Geometry check sheet. Reference: the model listing, model coordinates, mm. Face numbers are marked on the shaded views. A direction names the side the tool comes from. Give positions to 0.01 mm unless a question says otherwise; leave off trailing zeros. Order: outer loops, then holes, each group sorted by start corner. A loop starts at its lowest first (then second) coordinate and runs counter-clockwise, first axis right, second up. Notation, with made-up numbers: M 14.5,35.5 L 57.5,35.5 A32 cw 57.5,70.5 Z; hole C -15.75,30 d4. An arc over 180 degrees is marked long. Put each result on its own line as item: value. Start each with the question number.
Q1. Go/stop test with a flat-tipped pin: pin 1 (0.6 mm diameter, centred on x = 6.5, z = 1, fed in from -Y). Record where the tip stops, or that it passes through.
Q2. Section check B-B on z = 0.6. Record the cut outline in (x, y), then the cut area to 3 significant figures.
Q3. Material ranges on L1, parallel to Y at x = 3, z = 1.2; L2, parallel to X at y = 1.9, z = 0.2; L3, parallel to Z at x = 3.75, y = -0.4, recorded low to high.
Q4. Access from +Z, -Z, +X, -X, +Y, -Y to the whole of each face (thin tool, end or side, straight path). Record for the marked faces 1, 2, 3, 4 and 5.
Q5. Section check D-D on y = 2.45. Record the cut outline in (x, z), then the cut area to 3 significant figures.
Q6. Section check C-C on x = 4. Record the cut outline in (y, z).
Q7. Section check A-A on y = 3.1. Record the cut outline in (x, z).
```python
from build123d import *

# Parameters (mm, degrees)
SKETCH2_W            = 6.3
SKETCH2_H            = 2.6
BOSS_EXTRUDE1_DEPTH  = 1.4
EXTRUDE_THIN2_DEPTH  = 0.4
FILLET1_R            = 0.1
FILLET1_OF_MIRROR3_R = 0.1
MIRROR4_DEPTH        = 0.4
MIRROR4_START        = 2.2
MIRROR4_2_DEPTH      = 0.4
SKETCH4_W            = 0.2
SKETCH4_H            = 0.9
EXTRUDE_THIN3_DEPTH  = 0.2
SKETCH5_W            = 0.2
SKETCH5_H            = 0.9
EXTRUDE_THIN4_DEPTH  = 0.2
SKETCH6_W            = 0.2
SKETCH6_H            = 0.9
EXTRUDE_THIN5_DEPTH  = 0.2
SKETCH8_W            = 1.5
SKETCH8_H            = 1.1
BOSS_EXTRUDE2_DEPTH  = 1.5
FILLET2_R            = 0.2


# Read off the part's stored shape, not the designer's step: Mirror4
with BuildPart() as part:
    # Sketch2 → Boss-Extrude1 (new body)
    with BuildSketch(Plane.XY):
        with Locations((3.15, 1.3)):
            Rectangle(SKETCH2_W, SKETCH2_H)
    extrude(amount=BOSS_EXTRUDE1_DEPTH)

    # Sketch3 → Extrude-Thin2 (add)
    with BuildSketch(Plane.XZ):
        with BuildLine():
            Line((0, 1.4), (0, 0.3))
            ThreePointArc((0, 0.3), (-0.087867966, 0.087867966), (-0.3, 0))
            Line((-0.3, 0), (-0.7, 0))
            Line((-0.7, 0), (-0.7, 0.2))
            Line((-0.7, 0.2), (-0.3, 0.2))
            ThreePointArc((-0.3, 0.2), (-0.229289322, 0.229289322), (-0.2, 0.3))
            Line((-0.2, 0.3), (-0.2, 1.4))
            Line((-0.2, 1.4), (0, 1.4))
        make_face()
    extrude_thin2 = extrude(amount=-EXTRUDE_THIN2_DEPTH)

    # Fillet1
    fillet1_edges = [part.edges().sort_by_distance(p)[0] for p in [
        (-0.2, 0.2, 1.4),
    ]]
    fillet(fillet1_edges, radius=FILLET1_R)

    # Mirror3: Extrude-Thin2 across plane
    add(extrude_thin2.mirror(Plane.ZX.offset(1.3)))

    # Fillet1 of Mirror3
    fillet1_of_mirror3_edges = [part.edges().sort_by_distance(p)[0] for p in [
        (-0.2, 2.4, 1.4),
    ]]
    fillet(fillet1_of_mirror3_edges, radius=FILLET1_OF_MIRROR3_R)

    # Mirror4 outline → Mirror4 (add)
    with BuildSketch(Plane(origin=(0, 0, 0), x_dir=(1, 0, 0), z_dir=(0, 1, 0))):
        with BuildLine():
            Line((7, 0), (6.6, 0))
            ThreePointArc((6.6, 0), (6.387867966, -0.087867966), (6.3, -0.3))
            Line((6.3, -0.3), (6.3, -1.4))
            Line((6.3, -1.4), (6.4, -1.4))
            ThreePointArc((6.4, -1.4), (6.470710678, -1.370710678), (6.5, -1.3))
            Line((6.5, -1.3), (6.5, -0.3))
            ThreePointArc((6.5, -0.3), (6.529289322, -0.229289322), (6.6, -0.2))
            Line((6.6, -0.2), (7, -0.2))
            Line((7, -0.2), (7, 0))
        make_face()
    extrude(amount=MIRROR4_DEPTH)

    # Mirror4 2 outline → Mirror4 2 (add)
    with BuildSketch(Plane(origin=(0, 0, 0), x_dir=(1, 0, 0), z_dir=(0, 1, 0)).offset(MIRROR4_START)):
        with BuildLine():
            Line((7, 0), (6.6, 0))
            ThreePointArc((6.6, 0), (6.387867966, -0.087867966), (6.3, -0.3))
            Line((6.3, -0.3), (6.3, -1.4))
            Line((6.3, -1.4), (6.4, -1.4))
            ThreePointArc((6.4, -1.4), (6.470710678, -1.370710678), (6.5, -1.3))
            Line((6.5, -1.3), (6.5, -0.3))
            ThreePointArc((6.5, -0.3), (6.529289322, -0.229289322), (6.6, -0.2))
            Line((6.6, -0.2), (7, -0.2))
            Line((7, -0.2), (7, 0))
        make_face()
    extrude(amount=MIRROR4_2_DEPTH)

    # Sketch4 → Extrude-Thin3 (add, symmetric)
    with BuildSketch(Plane(origin=(0.9, 0, 0), x_dir=(0, 0, -1), z_dir=(1, 0, 0))):
        with Locations((-0.1, 3.05)):
            Rectangle(SKETCH4_W, SKETCH4_H)
    extrude(amount=EXTRUDE_THIN3_DEPTH, both=True)

    # Sketch5 → Extrude-Thin4 (add, symmetric)
    with BuildSketch(Plane(origin=(3.9, 0, 0), x_dir=(0, 0, -1), z_dir=(1, 0, 0))):
        with Locations((-0.1, 3.05)):
            Rectangle(SKETCH5_W, SKETCH5_H)
    extrude(amount=EXTRUDE_THIN4_DEPTH, both=True)

    # Sketch6 → Extrude-Thin5 (add, symmetric)
    with BuildSketch(Plane(origin=(5.4, 0, 0), x_dir=(0, 0, -1), z_dir=(1, 0, 0))):
        with Locations((-0.1, 3.05)):
            Rectangle(SKETCH6_W, SKETCH6_H)
    extrude(amount=EXTRUDE_THIN5_DEPTH, both=True)

    # Sketch8 → Boss-Extrude2 (add)
    with BuildSketch(Plane.XZ):
        with Locations((3.9, 0.65)):
            Rectangle(SKETCH8_W, SKETCH8_H)
    extrude(amount=BOSS_EXTRUDE2_DEPTH)

    # Fillet2
    fillet2_edges = [part.edges().sort_by_distance(p)[0] for p in [
        (3.15, -1.5, 0.65),
        (4.65, -1.5, 0.65),
    ]]
    fillet(fillet2_edges, radius=FILLET2_R)


solid = part.part
```
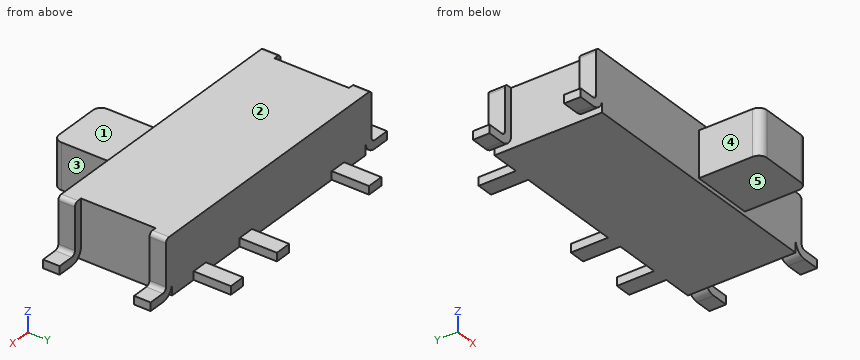
Results found:
1. pin 1: stops at y = 0
2. outline: M -0.2,0 L 3.15,0 L 3.15,-1.3 A0.2 ccw 3.35,-1.5 L 4.45,-1.5 A0.2 ccw 4.65,-1.3 L 4.65,0 L 6.5,0 L 6.5,0.4 L 6.3,0.4 L 6.3,2.2 L 6.5,2.2 L 6.5,2.6 L -0.2,2.6 L -0.2,2.2 L 0,2.2 L 0,0.4 L -0.2,0.4 Z
2. area: 18.9 mm^2
3. L1: y = 0 to 2.6
3. L2: x = 0 to 6.3
3. L3: z = 0.1 to 1.2
4. face 1: +Z, +X, -X, -Y
4. face 2: +Z, +X, -X, +Y, -Y
4. face 3: +Z, -Z, +X, -Y
4. face 4: +Z, -Z, -X, -Y
4. face 5: -Z, +X, -X, -Y
5. outline: M -0.7,0 L -0.3,0 A0.3 ccw 0,0.3 L 0,0 L 6.3,0 L 6.3,0.3 A0.3 ccw 6.6,0 L 7,0 L 7,0.2 L 6.6,0.2 A0.1 cw 6.5,0.3 L 6.5,1.3 A0.1 ccw 6.4,1.4 L -0.1,1.4 A0.1 ccw -0.2,1.3 L -0.2,0.3 A0.1 cw -0.3,0.2 L -0.7,0.2 Z
5. area: 9.54 mm^2
6. outline: M -1.5,0.1 L 0,0.1 L 0,0 L 3.5,0 L 3.5,0.2 L 2.6,0.2 L 2.6,1.4 L 0,1.4 L 0,1.2 L -1.5,1.2 Z
7. outline: M 0.7,0 L 1.1,0 L 1.1,0.2 L 0.7,0.2 Z; M 3.7,0 L 4.1,0 L 4.1,0.2 L 3.7,0.2 Z; M 5.2,0 L 5.6,0 L 5.6,0.2 L 5.2,0.2 Z
